Read the model definition and answer for the solid it produces. Units are mm, in the model's axes. A direction names the side the tool comes from. Give positions to 0.01 mm unless a question says otherwise; leave off trailing zeros. Loops run counter-clockwise (first coordinate to the right, second up) from the corner with the lowest first, then second, coordinate; pieces in that order, holes last. Notation, with made-up numbers: (23.5, 48) - (51.5, 48) arc R31 ccw to (51.5, 86) - close; hole circle Ø4 at (-29, 50.5). An arc over 180 degrees is marked (long way). Write item = value, one per line.
Autodesk Inventor part; units mm, degrees
ref_plane "YZ Plane" through (0, 0, 0) normal (1, 0, 0) x (0, 1, 0)
ref_plane "XZ Plane" through (0, 0, 0) normal (0, 1, 0) x (-1, 0, 0)
ref_plane "XY Plane" through (0, 0, 0) normal (0, 0, 1) x (1, 0, 0)
sketch "Эскиз1" plane through (0, 0, 0) normal (0, 1, 0) x (-1, 0, 0)
  line L0 (-25, -40) -> (25, -40)
  line L1 (25, -40) -> (25, 40)
  line L2 (25, 40) -> (-25, 40)
  line L3 (-25, 40) -> (-25, -40)
  line L4 (-25, -40) -> (25, 40) construction
  line L5 (25, -40) -> (-25, 40) construction
  line L6 (28, 43) -> (28, -43)
  line L7 (28, -43) -> (-28, -43)
  line L8 (-28, -43) -> (-28, 43)
  line L9 (-28, 43) -> (28, 43)
  line L10 (28, 43) -> (25, 43)
  line L11 (25, 43) -> (25, -43)
  line L12 (25, -43) -> (28, -43)
  line L13 (28, -43) -> (28, 43)
  line L14 (-28, 43) -> (-25, 43)
  line L15 (-25, 43) -> (-25, -43)
  line L16 (-25, -43) -> (-28, -43)
  line L17 (-28, -43) -> (-28, 43)
  point P0 (0, 0)
  point P1 (-25, 43)
  dimension "d0" = 50
  dimension "d1" = 80
  dimension "d2" = 3
extrude "Выдавливание1" add sketch "Эскиз1" along normal blind 1 contours L15 L7 L8 L9 L3 | L0 L11 L7 L15 | L1 L11 L9 L6 L7 | L15 L9 L11 L2
extrude "Выдавливание2" add sketch "Эскиз1" along normal blind 4 contours L15 L7 L8 L9 L3 | L0 L11 L7 L15 | L1 L11 L9 L6 L7
sketch "Эскиз2" plane through (-28, 0, 43) normal (0, 0, 1) x (1, 0, 0)
  line L0 (0, 0) -> (0, 4)
  line L1 (0, 1) -> (56, 1)
  line L2 (56, 0) -> (56, 4)
  line L3 (3, 0) -> (3, 4)
  line L4 (3, 4) -> (0.8, 1)
  line L5 (28, 0) -> (28, 4)
  line L6 (53, 4) -> (55.2, 1)
  line L7 (53, 0) -> (53, 4)
  line L8 (53, 4) -> (53, 1)
  point P0 (55.2, 1)
  point P1 (3, 1)
  dimension "d7" = 0.8
extrude "Выдавливание3" cut sketch "Эскиз2" against normal up to surface (83 mm away)
sketch "Эскиз3" plane through (-25, 0, -40) normal (0, 0, 1) x (1, 0, 0)
  line L0 (0, 0) -> (50, 0)
  line L1 (50, 0) -> (50, 1)
  line L2 (52.2, 1) -> (50, 1)
  line L3 (50, 4) -> (52.2, 1)
  line L4 (0, 4) -> (50, 4)
  line L5 (-2.2, 1) -> (0, 4)
  line L6 (0, 1) -> (-2.2, 1)
  line L7 (0, 0) -> (0, 1)
  line L8 (-2.2, 1) -> (52.2, 1)
  point P0 (25, 0)
extrude "Выдавливание4" cut sketch "Эскиз3" against normal blind 1 contours L6 L5 L4 L3 L2 L8
sketch "Эскиз4" plane through (28, 0, -43) normal (0, 0, -1) x (-1, 0, 0)
  line L0 (0, 0) -> (56, 0)
  line L1 (56, 0) -> (56, 4)
  line L2 (0, 4) -> (56, 4)
  line L3 (0, 0) -> (0, 4)
  point P0 (28, 0)
extrude "Выдавливание5" add sketch "Эскиз4" along normal blind 5
sketch "Эскиз5" plane through (-28, 0, 43) normal (0, 0, 1) x (1, 0, 0)
  line L0 (0.8, 1) -> (55.2, 1)
  line L1 (0.8, 1) -> (3, 4)
  line L2 (0, 4) -> (3, 4)
  line L3 (0, 0) -> (0, 4)
  line L4 (0, 0) -> (56, 0)
  line L5 (56, 0) -> (56, 4)
  line L6 (53, 4) -> (56, 4)
  line L7 (53, 4) -> (55.2, 1)
  point P0 (28, 0)
extrude "Выдавливание6" add sketch "Эскиз5" along normal blind 5
sketch "Эскиз6" plane through (-25, 0, -41) normal (0, 0, 1) x (1, 0, 0)
  line L0 (0, 4) -> (50, 4)
  line L1 (-2.2, 1) -> (0, 4)
  line L2 (52.2, 1) -> (-2.2, 1)
  line L3 (50, 4) -> (52.2, 1)
  point P0 (25, 0)
extrude "Выдавливание7" cut sketch "Эскиз6" against normal blind 3
sketch "Эскиз7" plane through (-28, 0, 48) normal (0, 0, 1) x (1, 0, 0)
  line L0 (56, 0) -> (56, 4)
  line L1 (56, 4) -> (53, 4)
  line L2 (53, 4) -> (55.2, 1)
  line L3 (55.2, 1) -> (0.8, 1)
  line L4 (0.8, 1) -> (3, 4)
  line L5 (3, 4) -> (0, 4)
  line L6 (0, 4) -> (0, 0)
  line L7 (0, 0) -> (56, 0)
  point P0 (28, 0)
extrude "Выдавливание8" add sketch "Эскиз7" along normal blind 7
sketch "Эскиз8" plane through (28, 0, -48) normal (0, 0, -1) x (-1, 0, 0)
  line L0 (0, 0) -> (56, 0)
  line L1 (56, 0) -> (56, 4)
  line L2 (56, 4) -> (0, 4)
  line L3 (0, 4) -> (0, 0)
  point P0 (28, 0)
extrude "Выдавливание9" add sketch "Эскиз8" along normal blind 7
sketch "Эскиз9" plane through (0, 4, 0) normal (0, 1, 0) x (1, 0, 0)
  line L0 (-28, -55) -> (-28, 55)
  line L1 (28, 55) -> (28, -55)
  line L2 (-28, 55) -> (28, 55)
  line L3 (28, 55) -> (28, 44)
  line L4 (28, 44) -> (-28, 44)
  line L5 (-28, 44) -> (-28, 55)
  line L6 (-28, 44) -> (28, 44)
  line L7 (28, 44) -> (28, 47)
  line L8 (28, 47) -> (-28, 47)
  line L9 (-28, 47) -> (-28, 44)
  point P0 (0, 0)
  point P1 (25, 44)
  dimension "d23" = 56
  dimension "d24" = 3
extrude "Выдавливание10" cut sketch "Эскиз9" against normal blind 2 contours L0 L2 L1 L8
fillet "Сопряжение2" radius 2 2 edges at (28, 1, -55) (-28, 1, -55)
fillet "Сопряжение3" radius 0.5 2 edges at (26.1, 2.5, 55) (-26.1, 2.5, 55)
properties part number "cover"
1) Each of these flat-tipped pins is pushed along its axis until it touches: P1, Ø0.6, axis at x = -11.5, y = 3, coming from the -Z side; P2, Ø2, axis at x = -22.5, z = -35.5, coming from the -Y side; P3, Ø4, axis at x = 1, z = -51.5, coming from the +Y side. Where does it stop, or does it pass through?
Output:
P1 = -47
P2 = through
P3 = 2
2) A cutting plane is placed at A-A on x = 13. Determine the outline of the cut face in (y, z), then the cut area to 3 significant figures.
Output:
outline = (0, -55) - (2, -55) - (2, -47) - (4, -47) - (4, -44) - (1, -44) - (1, -40) - (0, -40) - close; (0, 40) - (1, 40) - (1, 55) - (0, 55) - close
area = 47.0 mm²
3) A tool of negligible diameter and unlimited length cuts with its end or side. For faces 1 (the face through (0, 2, -51)), 2 (the face through (-28, 2, 2)), from which of +Z, -Z, +X, -X, +Y, -Y can it reach the whole face along a straight path? Write none if from no direction.
Output:
face_1 = -Z, +X, -X, +Y
face_2 = +Z, -Z, -X, +Y, -Y
4) Find the intervals of material crossed by probe 1 along X at (y, z) = (2.65, -3); probe 2 along Y at (x, z) = (18.5, -47.5); probe 3 along X at (y, z) = (0.55, 15.5), in increasing order.
Output:
probe_1 = -28 to -25.99, 25.99 to 28
probe_2 = 0 to 2
probe_3 = -28 to -25, 25 to 28
5) A cutting plane is placed at B-B on z = -28. Determine the outline of the cut face in (x, y), then the cut area to 3 significant figures.
Output:
outline = (-28, 0) - (-25, 0) - (-25, 1) - (-27.2, 1) - (-25, 4) - (-28, 4) - close; (25, 0) - (28, 0) - (28, 4) - (25, 4) - (27.2, 1) - (25, 1) - close
area = 17.4 mm²
6) The mould has two halves that part along Y. Classify faces 3 (the face through (-27, 4, -7)), 4 (the face through (28, 2, 2)), 5 (the face through (26.1, 2.5, 4.6)): pulls with the +Y half, pulls with the -Y half, needs draft (parallel to the pull), parting line crosses it, or undercut.
Output:
face_3 = pulls with the +Y half
face_4 = needs draft
face_5 = undercut
